Part model, mm, in its own coordinate system. Give positions to 0.01 mm unless a question says otherwise; leave off trailing zeros. Order: outer loops, then holes, each group sorted by start corner. A loop starts at its lowest first (then second) coordinate and runs counter-clockwise, first axis right, second up. Notation, with made-up numbers: M 75.5,19.5 L 95.5,19.5 A21 ccw 95.5,53.5 Z; hole C -27,35.5 d9. An arc over 180 degrees is marked long. Answer as a JSON object with one key per item and string values.
from build123d import *

# Parameters (mm, degrees)
SKETCH5_R = 1.524


with BuildPart() as part:
    # Sweep1: sweep along a path in Sketch1
    with BuildLine(Plane.XY) as sweep1_path:
        Line((-67.31, -9.652), (-67.31, -1.524))
        ThreePointArc((-67.31, -1.524), (-66.863630735, -0.446369265), (-65.786, 0))
        Line((-65.786, 0), (65.786, 0))
        ThreePointArc((65.786, 0), (66.863630735, -0.446369265), (67.31, -1.524))
        Line((67.31, -1.524), (67.31, -9.652))
    # Sketch5 → Sweep1 (sweep)
    with BuildSketch(Plane(origin=(0, -9.652, 0), x_dir=(-1, 0, 0), z_dir=(0, 1, 0))):
        with Locations((67.31, 0)):
            Circle(SKETCH5_R)
    sweep(path=sweep1_path.line)


solid = part.part
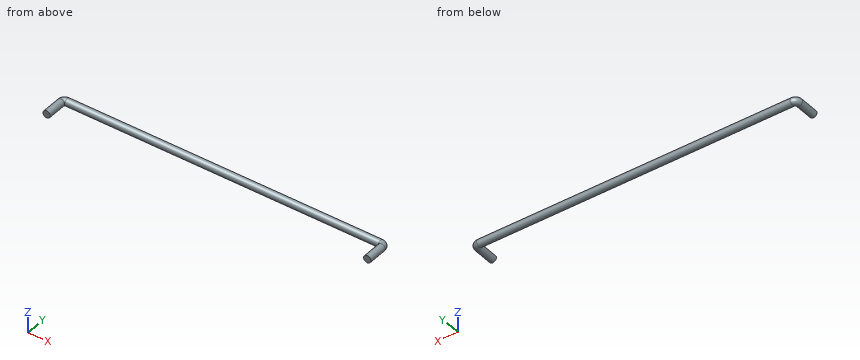
1. Cut at B-B on x = 43.5. Give the cut face in (y, z), plus the area to 3 significant figures.
Worked answers:
{"outline": "C 0,0 d3.05", "area": "7.30 mm^2"}
2. Probe line 1 along X through (y, z) = (-7.5, -0.8); line 2 along X through (y, z) = (-3.75, -0.55); line 3 along Y through (x, z) = (-26.5, 0.15). List the from-to ranges inside material, lowest first.
Worked answers:
{"line 1": "x = -68.61 to -66.01, 66.01 to 68.61", "line 2": "x = -68.73 to -65.89, 65.89 to 68.73", "line 3": "y = -1.52 to 1.52"}
3. Pin check, flat tips, straight feed: P1, Ø5, axis at x = 21, y = -3, coming from the +Z side; P2, Ø1.5, axis at y = -7, z = 1, coming from the +X side. Stop position of each tip, or through.
Worked answers:
{"P1": "stops at z = 1.44", "P2": "stops at x = 68.81"}
4. Cut at A-A on y = -4.75. Give the cut face in (x, z).
Worked answers:
{"outline": "C -67.31,0 d3.05; C 67.31,0 d3.05"}
